Can you work these out from the model? Positions are in its coordinate system, mm. Face numbers are marked on the shaded views. A direction names the side the tool comes from. Round coordinates to 2 decimals unless told otherwise and drop trailing zeros. Loops run counter-clockwise (first coordinate to the right, second up) from the corner with the lowest first, then second, coordinate; pieces in that order, holes last. Notation, with made-up numbers: M 26.5,50 L 74.5,50 A35 ccw 74.5,86 Z; hole C 67.25,75 d5. An arc over 180 degrees is marked long. Use a Markdown table: item, result. Add a question column.
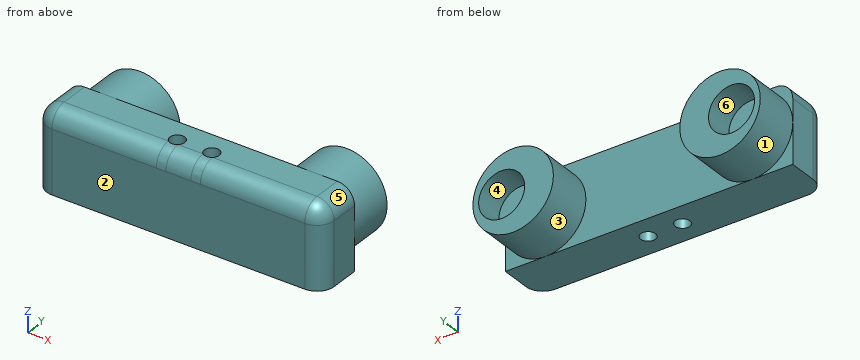
```python
from build123d import *

# Parameters (mm, degrees)
SKETCH_W     = 50
SKETCH_H     = 8
SKETCH_R     = 1.3
PAD_DEPTH    = 14
SKETCH001_R  = 7
PAD001_DEPTH = 8
SKETCH002_R  = 4
POCKET_DEPTH = 5
FILLET_R     = 3


with BuildPart() as part:
    # Sketch → Pad (new body)
    with BuildSketch(Plane.XY):
        with Locations((-25, 4)):
            Rectangle(SKETCH_W, SKETCH_H)
        with Locations((-28, 4)):
            Circle(SKETCH_R, mode=Mode.SUBTRACT)
        with Locations((-22, 4)):
            Circle(SKETCH_R, mode=Mode.SUBTRACT)
    extrude(amount=PAD_DEPTH)

    # Sketch001 (on Face1 of Pad) → Pad001 (join)
    with BuildSketch(Plane(origin=(0, 8, 0), x_dir=(-1, 0, 0), z_dir=(0, 1, 0))):
        with Locations((7, 7)):
            Circle(SKETCH001_R)
        with Locations((43, 7)):
            Circle(SKETCH001_R)
    extrude(amount=PAD001_DEPTH)

    # Sketch002 (on Face5 of Pad001) → Pocket (cut)
    with BuildSketch(Plane(origin=(0, 16, 0), x_dir=(-1, 0, 0), z_dir=(0, 1, 0))):
        with Locations((5, 7)):
            Circle(SKETCH002_R)
        with Locations((45, 7)):
            Circle(SKETCH002_R)
    extrude(amount=-POCKET_DEPTH, mode=Mode.SUBTRACT)

    # Fillet
    fillet_edges = [part.edges().sort_by_distance(p)[0] for p in [
        (0, 0, 7),
        (-25, 0, 14),
        (-50, 0, 7),
        (0, 4, 14),
        (-50, 4, 14),
    ]]
    fillet(fillet_edges, radius=FILLET_R)


solid = part.part
```
(1) Suppose I cut it at C-C on x = -35. List the corners of the cut face in (y, z) for me.
(2) I'm going to push flat-ended pins straight in: pin 1 (6.5 mm diameter, centred on x = -45, z = 7, fed in from +Y); pin 2 (1.5 mm diameter, centred on y = 10.5, z = 9.5, fed in from -X). Where does each tip first touch, or does it pass through?
(3) If I drill on probe 1 along X at (y, z) = (4, 10.25); probe 2 along Y at (x, z) = (-22, 3); probe 3 along X at (y, z) = (4.5, 2.5), over which ranges is the centre line in solid material (lowest first)? Write a range as [from, to].
(4) Suppose I cut it at A-A on y = 13.5. List the corners of the cut face in (x, z) for me.
(5) On a 3-axis mill with a long thin cutter (end or side, diameter ignored), from which of +Z, -Z, +X, -X, +Y, -Y can I reach the whole of each face in a straight line? I mean the marked faces 1 and 2. Say none if no direction works.
(6) Suppose I cut it at D-D on z = 6.25. List the corners of the cut face in (x, y) for me.
(7) Thinking about a two-plate mould opening in Z: for the marked faces 3, 4, 5 and 6, which applies, released by +Z, released by -Z, zero draft, split by the parting line, or undercut?
(8) Suppose I cut it at B-B on z = 8.75. List the corners of the cut face in (x, y) for me.
Results below:
| question | item | result |
|---|---|---|
| 1 | outline | M 0,0 L 8,0 L 8,14 L 3,14 A3 ccw 0,11 Z |
| 2 | pin 1 | stops at y = 11 |
| 2 | pin 2 | stops at x = -49.78 |
| 3 | probe 1 | x = [-50, -29.3], [-26.7, -23.3], [-20.7, 0] |
| 3 | probe 2 | y = [0, 2.7], [5.3, 8] |
| 3 | probe 3 | x = [-50, -29.2], [-26.8, -23.2], [-20.8, 0] |
| 4 | outline | C -43,7 d14; C -7,7 d14; hole C -45,7 d8; hole C -5,7 d8 |
| 5 | face 1 | +Y |
| 5 | face 2 | +Z, -Z, +X, -X, -Y |
| 6 | outline | M -50,3 A3 ccw -47,0 L -3,0 A3 ccw 0,3 L 0,8 L -0.04,8 L -0.04,16 L -1.07,16 L -1.07,11 L -8.93,11 L -8.93,16 L -13.96,16 L -13.96,8 L -36.04,8 L -36.04,16 L -41.07,16 L -41.07,11 L -48.93,11 L -48.93,16 L -49.96,16 L -49.96,8 L -50,8 Z; hole C -28,4 d2.6; hole C -22,4 d2.6 |
| 7 | face 3 | split by the parting line |
| 7 | face 4 | undercut |
| 7 | face 5 | released by +Z |
| 7 | face 6 | undercut |
| 8 | outline | M -50,3 A3 ccw -47,0 L -3,0 A3 ccw 0,3 L 0,8 L -0.22,8 L -0.22,16 L -1.4,16 L -1.4,11 L -8.6,11 L -8.6,16 L -13.78,16 L -13.78,8 L -36.22,8 L -36.22,16 L -41.4,16 L -41.4,11 L -48.6,11 L -48.6,16 L -49.78,16 L -49.78,8 L -50,8 Z; hole C -28,4 d2.6; hole C -22,4 d2.6 |
